from build123d import *

# Parameters (mm, degrees)
F1_DEPTH = 20
F2_R     = 1.65
F3_DEPTH = 7.201
F5_DEPTH = 9
F7_DEPTH = 4
F9_DEPTH = 16.001


with BuildPart() as f1:
    # F0 (on Front) → F1 (new body)
    with BuildSketch(Plane.XZ):
        Polygon((-4, 0), (0, 0), (4, 0), (4, 1), (6.5, 1), (6.5, 2), (2.75, 7.2), (0, 7.2), (-2.75, 7.2), (-6.5, 2), (-6.5, 1), (-4, 1), align=None)
    extrude(amount=F1_DEPTH)

    # F2 (on face) → F3 (cut, through all)
    with BuildSketch(Plane(origin=(0, 0, 0), x_dir=(1, 0, 0), z_dir=(0, 0, -1))):
        with Locations((0, 14)):
            Circle(F2_R)
    extrude(amount=-F3_DEPTH, mode=Mode.SUBTRACT)

    # F4 (on Front) → F5 (join)
    with BuildSketch(Plane.XZ):
        with BuildLine():
            Line((1.6124515497, 7.2), (2.75, 7.2))
            ThreePointArc((2.75, 7.2), (0, 9), (-2.75, 7.2))
            Line((-2.75, 7.2), (-1.6124515497, 7.2))
            ThreePointArc((-1.6124515497, 7.2), (0, 8.2), (1.6124515497, 7.2))
        make_face()
    extrude(amount=F5_DEPTH)

    # F6 (on face) → F7 (cut)
    with BuildSketch(Plane(origin=(0, 0, 0), x_dir=(-1, 0, 0), z_dir=(0, 1, 0))):
        with BuildLine():
            ThreePointArc((2.75, 7.2), (0, 9), (-2.75, 7.2))
            Line((-2.75, 7.2), (-1.6124515497, 7.2))
            ThreePointArc((-1.6124515497, 7.2), (0, 8.2), (1.6124515497, 7.2))
            Line((1.6124515497, 7.2), (2.75, 7.2))
        make_face()
    extrude(amount=-F7_DEPTH, mode=Mode.SUBTRACT)

    # F8 (on face) → F9 (cut, through all)
    with BuildSketch(Plane(origin=(0, -4, 0), x_dir=(-1, 0, 0), z_dir=(0, 1, 0))):
        with BuildLine():
            Line((-0.25, 8.9895676091), (-0.25, 8.182554347))
            ThreePointArc((-0.25, 8.182554347), (0, 8.2), (0.25, 8.182554347))
            Line((0.25, 8.182554347), (0.25, 8.9895676091))
            ThreePointArc((0.25, 8.9895676091), (0, 9), (-0.25, 8.9895676091))
        make_face()
    extrude(amount=-F9_DEPTH, mode=Mode.SUBTRACT)


solid = f1.part
Input: part model. Units: mm. Frame: model coordinates. A direction names the side the tool comes from. Coordinates: 2 decimals unless noted, no trailing zeros. Loops run counter-clockwise (first coordinate to the right, second up) from the corner with the lowest first, then second, coordinate; pieces in that order, holes last.
Q1. Cut plane D-D (z = 6). Output: boundary loops of the cut face in (x, y).
Q2. Set-up query: faces 5 (the face through (-1.5, -4, 8.1)), 6 (the face through (-4, -9.9, 0.5)), 7 (the face through (0.25, -6.5, 8.6)), 8 (the face through (5, -10, 1)), 9 (the face through (1.5, -9, 8.1)). Return all of +Z, -Z, +X, -X, +Y, -Y with unobstructed straight access to the full face (end or side cutting, diameter ignored); none if empty.
Q3. Material intervals for line 1 (Y direction, x = 0, z = 5.5); line 2 (X direction, y = -14, z = 1.5); line 3 (X direction, y = -14, z = 4.5), sorted ascending.
Q4. Cut plane B-B (x = 0). Output: boundary loops of the cut face in (y, z).
Q5. Contact query for flat-ended pins moving along their axis: pin 1 (0.5 mm diameter, centred on y = -11, z = 0.5, fed in from +X); pin 2 (4 mm diameter, centred on x = 2.5, y = -9.5, fed in from +Z); pin 3 (1.4 mm diameter, centred on x = -2, z = 8, fed in from +Y). Output: stop coordinate, or through.
Q6. Draft query along Z for faces 1 (the face through (-4.599, -9.86, 4.636)), 2 (the face through (2, -4, 8)), 3 (the face through (-5, -10, 1)), 4 (the face through (-1.063, -6.465, 7.853)). Return one class per face: +Z half, -Z half, draft (parallel to the pull), parting line (faces both ways), or undercut.
Q7. Cut plane C-C (y = -2.25). Output: boundary loops of the cut face in (x, z).
Q8. Cut plane A-A (y = -14). Output: boundary loops of the cut face in (x, z), then the cut area to 3 significant figures.
Working result:
1. outline: (-3.62, -20) - (3.62, -20) - (3.62, 0) - (-3.62, 0) - close; hole circle Ø3.3 at (0, -14)
2. face 5: +Z, +X, -X, +Y
2. face 6: -Z, -X, +Y, -Y
2. face 7: +Z, +Y, -Y
2. face 8: -Z, +X, +Y, -Y
2. face 9: +Z, +X, -X, -Y
3. line 1: y = -20 to -15.65, -12.35 to 0
3. line 2: x = -6.5 to -1.65, 1.65 to 6.5
3. line 3: x = -4.7 to -1.65, 1.65 to 4.7
4. outline: (-20, 0) - (-15.65, 0) - (-15.65, 7.2) - (-20, 7.2) - close; (-12.35, 0) - (0, 0) - (0, 7.2) - (-12.35, 7.2) - close
5. pin 1: stops at x = 4
5. pin 2: stops at z = 8.95
5. pin 3: stops at y = -4
6. face 1: +Z half
6. face 2: draft
6. face 3: -Z half
6. face 4: undercut
7. outline: (-6.5, 1) - (-4, 1) - (-4, 0) - (4, 0) - (4, 1) - (6.5, 1) - (6.5, 2) - (2.75, 7.2) - (-2.75, 7.2) - (-6.5, 2) - close
8. outline: (-6.5, 1) - (-4, 1) - (-4, 0) - (-1.65, 0) - (-1.65, 7.2) - (-2.75, 7.2) - (-6.5, 2) - close; (1.65, 0) - (4, 0) - (4, 1) - (6.5, 1) - (6.5, 2) - (2.75, 7.2) - (1.65, 7.2) - close
8. area: 45.3 mm2
